```python
from build123d import *

# Parameters (mm, degrees)
CROQUIS1_R                 = 1.5
CROQUIS1_W                 = 3
CROQUIS1_H                 = 7.999999999
CROQUIS1_H_2               = 5
SALIENTE_EXTRUIR1_DEPTH    = 3
S_LIDO_MOVER_COPIAR1_ANGLE = 90


with BuildPart() as part:
    # Croquis1 → Saliente-Extruir1 (new body)
    with BuildSketch(Plane.XY):
        with BuildLine():
            Line((41807.173257962, -434.43949549), (41807.173257962, -346.219921492))
            ThreePointArc((41807.173257962, -346.219921492), (41801.173257962, -331.699124202), (41795.173257962, -346.219921492))
            Line((41795.173257962, -346.219921492), (41795.173257962, -434.43949549))
            ThreePointArc((41795.173257962, -434.43949549), (41801.173257962, -440.43949549), (41807.173257962, -434.43949549))
        make_face()
        with Locations((41801.173257962, -337.699124202)):
            Circle(CROQUIS1_R, mode=Mode.SUBTRACT)
        with Locations((41801.173257962, -403.93949549)):
            Circle(CROQUIS1_R, mode=Mode.SUBTRACT)
        with Locations((41801.173257962, -436.93949549)):
            Circle(CROQUIS1_R, mode=Mode.SUBTRACT)
        with Locations((41801.173257962, -369.439495491)):
            Rectangle(CROQUIS1_W, CROQUIS1_H, mode=Mode.SUBTRACT)
        with Locations((41801.173257962, -422.93949549)):
            Rectangle(CROQUIS1_W, CROQUIS1_H_2, mode=Mode.SUBTRACT)
    extrude(amount=SALIENTE_EXTRUIR1_DEPTH)


with BuildPart() as part_1:
    # Sólido-Mover/Copiar1: moved
    add(part.part.rotate(Axis((0, -386.069309846, 1.5), (-1, 0, 0)), S_LIDO_MOVER_COPIAR1_ANGLE))


solid = part_1.part
```
Part model, mm, in its own coordinate system. A direction names the side the tool comes from. Coordinates: 2 decimals unless noted, no trailing zeros. Order: outer loops, then holes, each group sorted by start corner. A loop starts at its lowest first (then second) coordinate and runs counter-clockwise, first axis right, second up. Notation, with made-up numbers: (-11.75, 28.25) - (33.25, 28.25) arc R3 cw to (33.25, 33.25) - close; hole circle Ø1 at (29, -30). An arc over 180 degrees is marked (long way). Return JSON: item names as keys, results as strings. Group by question number.
Item 1: Drill centre lines: probe 1 along Z at (x, y) = (41801.5, -386.8); probe 2 along X at (y, z) = (-386.35, 24); probe 3 along Z at (x, y) = (41802, -385.05). Where is each one in solid material? Low to high. Write a range as from..to.
Item 2: Pull direction Z, two halves, no side cores. Call faces 4 (the face through (41801.04, -386.09, 55.87)), 5 (the face through (41795.173, -386, 5)), 6 (the face through (41801.454, -386.09, -52.866)), 7 (the face through (41802.56, -386.09, 52.94)): pulls with the +Z half, pulls with the -Z half, needs draft (parallel to the pull), parting line crosses it, or undercut.
Item 3: Cut at A-A (y = -386.65). List the corners of the cut face in (x, z).
Item 4: Cut at C-C (x = 41806.25). List the corners of the cut face in (y, z), plus the area to 3 significant figures.
Item 5: Which spindle directions (+Z, -Z, +X, -X, +Y, -Y) get a long thin tool onto all of the face, cutting with end or side? Do faces 1 (the face through (41807.173, -386, 6)), 2 (the face through (41801, -384.569, 1)), 3 (the face through (41799.673, -386, 38)). Say none if no direction does.
Item 6: Pin check, flat tips, straight feed: pin 1 (3.5 mm diameter, centred on x = 41801.17, z = -46.87, fed in from +Y); pin 2 (0.9 mm diameter, centred on y = -386.5, z = -16, fed in from +X); pin 3 (0.9 mm diameter, centred on y = -386, z = -14.5, fed in from -X); pin 4 (1 mm diameter, centred on x = 41796.5, y = -387, fed in from +Z). Stop position of each tip, or through.
Item 7: Cut at B-B (z = -6.5). List the corners of the cut face in (x, y).
Check values:
{
 "1": {"probe 1": "z = -52.86..-48.33, -45.41..-19.13, -11.13..17.91, 20.83..35.87, 40.87..50.91, 53.83..55.86", "probe 2": "x = 41795.17..41807.17", "probe 3": "z = -52.83..-48.12, -45.62..-19.13, -11.13..18.12, 20.62..35.87, 40.87..51.12, 53.62..55.81"},
 "2": {"face 4": "pulls with the +Z half", "face 5": "needs draft", "face 6": "parting line crosses it", "face 7": "undercut"},
 "3": {"outline": "(41795.17, -38.35) arc R8.5 ccw (long way) to (41807.17, -38.35) - (41807.17, 49.87) arc R6 ccw to (41795.17, 49.87) - close; hole circle Ø3 at (41801.17, -46.87); hole (41799.67, -19.13) - (41802.67, -19.13) - (41802.67, -11.13) - (41799.67, -11.13) - close; hole circle Ø3 at (41801.17, 19.37); hole (41799.67, 35.87) - (41802.67, 35.87) - (41802.67, 40.87) - (41799.67, 40.87) - close; hole circle Ø3 at (41801.17, 52.37)"},
 "4": {"outline": "(-387.57, -51.19) - (-384.57, -51.19) - (-384.57, 53.07) - (-387.57, 53.07) - close", "area": "313 mm2"},
 "5": {"face 1": "+Z, +X, +Y, -Y", "face 2": "+Z, -Z, +X, -X, +Y", "face 3": "+Y, -Y"},
 "6": {"pin 1": "stops at y = -384.57", "pin 2": "stops at x = 41807.17", "pin 3": "stops at x = 41795.17", "pin 4": "stops at z = 54.18"},
 "7": {"outline": "(41795.17, -387.57) - (41807.17, -387.57) - (41807.17, -384.57) - (41795.17, -384.57) - close"}
}
